The figure shows three views and two pictorial views of one solid part (mm, origin at its lowest corner). Answer the questions. A direction names the side the tool comes from. Give positions to 0.01 mm unless a question says otherwise; leave off trailing zeros. Write each loop counter-clockwise with the first axis right and the second up, starting at its lowest first coordinate (ties: lowest second). Pieces come first, ordered by that corner, then holes. Notation, with made-up numbers: (9, 57) - (30, 57) arc R24 cw to (30, 76) - close; hole circle Ø11 at (-12.75, 0.5). An arc over 180 degrees is marked (long way). Use a Markdown table: item, result. Add a question column.
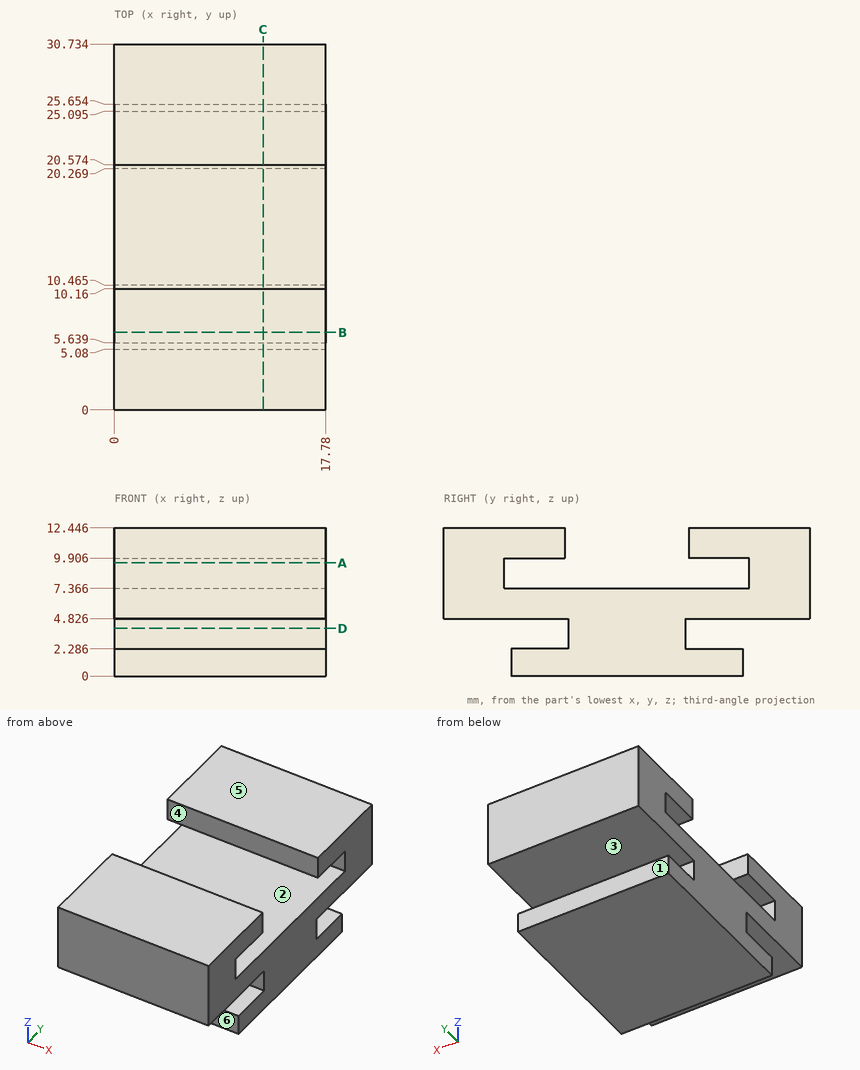
1. Given P1, Ø1.8, axis at x = 6.5, z = 1, coming from the +Y side (3 decimals); P2, Ø1.1, axis at x = 10, z = 0.5, coming from the -Y side, each flat-ended and moving along its own axis, determine where each tip first touches the part or whether it passes through.
2. The part is cut by section C-C (x = 12.5). Give the vertices of the cut face in (y, z) (1 decimal), and give its area (3 significant figures).
3. The part is cut by section D-D (z = 4). Give the vertices of the cut face in (x, y) (1 decimal).
4. For a pull along Y with two mould halves and no side action, classify the marked faces 4, 5 and 6 as released by +Y, released by -Y, zero draft, split by the parting line, or undercut.
5. Consider L1, parallel to Z at x = 5.5, y = 23; L2, parallel to Y at x = 1, z = 11.75; L3, parallel to Y at x = 1, z = 9.5. Determine where each line is inside the solid, lowest interval first. Write a range as [from, to].
6. Which of the six approach directions +Z, -Z, +X, -X, +Y, -Y give full straight-line access (tool end or side, diameter ignored) to the marked faces 1, 2 and 3?
7. The part is cut by section B-B (y = 6.5). Give the vertices of the cut face in (x, z).
8. The part is cut by section A-A (z = 9.5). Give the vertices of the cut face in (x, y), and give its area (3 significant figures).
Check values:
| question | item | result |
|---|---|---|
| 1 | P1 | stops at y = 25.095 |
| 1 | P2 | stops at y = 5.64 |
| 2 | outline | (0, 4.8) - (10.5, 4.8) - (10.5, 2.3) - (5.6, 2.3) - (5.6, 0) - (25.1, 0) - (25.1, 2.3) - (20.3, 2.3) - (20.3, 4.8) - (30.7, 4.8) - (30.7, 12.4) - (20.6, 12.4) - (20.6, 9.9) - (25.7, 9.9) - (25.7, 7.4) - (5.1, 7.4) - (5.1, 9.9) - (10.2, 9.9) - (10.2, 12.4) - (0, 12.4) - close |
| 2 | area | 225 mm2 |
| 3 | outline | (0, 10.5) - (17.8, 10.5) - (17.8, 20.3) - (0, 20.3) - close |
| 4 | face 4 | undercut |
| 4 | face 5 | zero draft |
| 4 | face 6 | released by -Y |
| 5 | L1 | z = [0, 2.29], [4.83, 7.37], [9.91, 12.45] |
| 5 | L2 | y = [0, 10.16], [20.57, 30.73] |
| 5 | L3 | y = [0, 5.08], [25.65, 30.73] |
| 6 | face 1 | -Z, +X, -X, +Y |
| 6 | face 2 | +X, -X |
| 6 | face 3 | +X, -X, +Y |
| 7 | outline | (0, 0) - (17.78, 0) - (17.78, 2.29) - (0, 2.29) - close; (0, 4.83) - (17.78, 4.83) - (17.78, 7.37) - (0, 7.37) - close; (0, 9.91) - (17.78, 9.91) - (17.78, 12.45) - (0, 12.45) - close |
| 8 | outline | (0, 0) - (17.78, 0) - (17.78, 5.08) - (0, 5.08) - close; (0, 25.65) - (17.78, 25.65) - (17.78, 30.73) - (0, 30.73) - close |
| 8 | area | 181 mm2 |
